Input: part model. Units: mm. Frame: model coordinates. A direction names the side the tool comes from. Coordinates: 2 decimals unless noted, no trailing zeros. Write each loop counter-clockwise with the first axis right and the second up, starting at its lowest first coordinate (ties: lowest second). Pieces come first, ordered by that corner, then holes. Notation, with made-up numbers: M 3.5,-13 L 54.5,-13 A37 ccw 54.5,26 Z; hole C 38,85 d3. An arc over 180 degrees is marked long. Use one line per item in the form item = value.
from build123d import *

# Parameters (mm, degrees)
CROQUIS1_W              = 240
CROQUIS1_H              = 14
SALIENTE_EXTRUIR2_DEPTH = 3
CROQUIS3_R              = 4.466306423
CROQUIS3_R_2            = 3.970050153
CORTAR_EXTRUIR1_DEPTH   = 1.3
CROQUIS4_R              = 0.75
CORTAR_EXTRUIR2_DEPTH   = 121.851148112


with BuildPart() as part:
    # Croquis1 → Saliente-Extruir2 (new body)
    with BuildSketch(Plane(origin=(0, 0, 0), x_dir=(1, 0, 0), z_dir=(0, 1, 0))):
        Rectangle(CROQUIS1_W, CROQUIS1_H)
    extrude(amount=SALIENTE_EXTRUIR2_DEPTH)

    # Croquis3 → Cortar-Extruir1 (cut)
    with BuildSketch(Plane(origin=(0, 3, 0), x_dir=(1, 0, 0), z_dir=(0, 1, 0))):
        with Locations(Location((-89.977775034, -2, 0), (0, 0, 270))):
            Circle(CROQUIS3_R)
        with Locations(Location((89.977775034, -2, 0), (0, 0, 270))):
            Circle(CROQUIS3_R_2)
    extrude(amount=-CORTAR_EXTRUIR1_DEPTH, mode=Mode.SUBTRACT)

    # Croquis4 → Cortar-Extruir2 (cut, through all)
    with BuildSketch(Plane(origin=(0, 0, -7), x_dir=(-1, 0, 0), z_dir=(0, 0, -1))):
        with Locations((-110, 1.5)):
            Circle(CROQUIS4_R)
        with Locations(Location((110, 1.5, 0), (0, 0, 180))):
            Circle(CROQUIS4_R)
    extrude(amount=-CORTAR_EXTRUIR2_DEPTH, mode=Mode.SUBTRACT)


solid = part.part
(1) First-contact query: pin 1 Ø2.5 at (x, z) = (-90.5, 2) entering from +Y. Flat tip, straight axial feed; report the tip coordinate or a pass-through.
Computed:
pin_1 = 1.7
(2) Section query A-A on z = 2. Return the cut outline in (x, y), plus the area to 3 significant figures.
Computed:
outline = M -120,0 L 120,0 L 120,3 L 93.95,3 L 93.95,1.7 L 86.01,1.7 L 86.01,3 L -85.51,3 L -85.51,1.7 L -94.44,1.7 L -94.44,3 L -120,3 Z; hole C -110,1.5 d1.5; hole C 110,1.5 d1.5
area = 695 mm^2
(3) Line query: probe 1 along X at (y, z) = (2.35, 2); probe 2 along X at (y, z) = (1.4, 2); probe 3 along X at (y, z) = (1.9, 1). Output: solid intervals per line, ascending.
Computed:
probe_1 = -120 to -94.44, -85.51 to 86.01, 93.95 to 120
probe_2 = -120 to -110.74, -109.26 to 109.26, 110.74 to 120
probe_3 = -120 to -110.63, -109.37 to -94.33, -85.62 to 86.14, 93.82 to 109.37, 110.63 to 120
(4) Pull-direction query (X, two-part tool) for faces 3 (the flat face through (-2, 3, 0)), 4 (the flat face through (90, 1.7, 2)); classes: pulls with the +X half, pulls with the -X half, needs draft (parallel to the pull), parting line crosses it, or undercut.
Computed:
face_3 = needs draft
face_4 = undercut
(5) Set-up query: faces 1 (the flat face through (-2, 0, 0)), 2 (the cylindrical face through (-94.338, 2.359, 1.032)). Return all of +Z, -Z, +X, -X, +Y, -Y with unobstructed straight access to the full face (end or side cutting, diameter ignored); none if empty.
Computed:
face_1 = +Z, -Z, +X, -X, -Y
face_2 = +Y
